```python
from build123d import *

# Parameters (mm, degrees)
EXTRUDE1_DEPTH                                       = 12.7
EXTRUDE2_DEPTH                                       = 3.175
SKETCH3_W                                            = 68.191134733
SKETCH3_H                                            = 44.45
EXTRUDE3_DEPTH                                       = 3.175
SKETCH4_W                                            = 68.191134733
SKETCH4_H                                            = 19.005533376
EXTRUDE4_DEPTH                                       = 3.175
EXTRUDE6_DEPTH                                       = 137.930502446
CBORE_FOR_1_4_BINDING_HEAD_MACHINE_SCREW_D           = 9.525
CBORE_FOR_1_4_BINDING_HEAD_MACHINE_SCREW_CBORE_D     = 17.4752
CBORE_FOR_1_4_BINDING_HEAD_MACHINE_SCREW_CBORE_DEPTH = 3.175
F_7_32_0_21875_DIAMETER_HOLE1_D                      = 5.55625
F_7_32_0_21875_DIAMETER_HOLE1_DEPTH                  = 25.4
F_7_32_0_21875_DIAMETER_HOLE1_TIP                    = 1.669265907
F_7_32_0_21875_DIAMETER_HOLE2_D                      = 5.55625
F_7_32_0_21875_DIAMETER_HOLE2_DEPTH                  = 25.4
F_7_32_0_21875_DIAMETER_HOLE2_TIP                    = 1.669265907


with BuildPart() as part:
    # Sketch1 → Extrude1 (new body)
    with BuildSketch(Plane(origin=(0, 0, 0), x_dir=(1, 0, 0), z_dir=(0, 1, 0))):
        with BuildLine():
            Line((0, 0), (101.6, 0))
            ThreePointArc((101.6, 0), (127, 25.4), (101.6, 50.8))
            Line((101.6, 50.8), (0, 50.8))
            ThreePointArc((0, 50.8), (-24.665230296, 25.4), (0, 0))
        make_face()
    extrude(amount=-EXTRUDE1_DEPTH)

    # Sketch2 → Extrude2 (cut)
    with BuildSketch(Plane(origin=(0, 0, 0), x_dir=(1, 0, 0), z_dir=(0, 1, 0))):
        with BuildLine():
            Line((101.6, 47.625), (0.048151693, 47.625))
            ThreePointArc((0.048151693, 47.625), (-21.490230296, 25.4), (0.048151693, 3.175))
            Line((0.048151693, 3.175), (101.6, 3.175))
            ThreePointArc((101.6, 3.175), (123.825, 25.4), (101.6, 47.625))
        make_face()
    extrude(amount=-EXTRUDE2_DEPTH, mode=Mode.SUBTRACT)

    # Sketch3 → Extrude3 (cut)
    with BuildSketch(Plane(origin=(0, -3.175, 0), x_dir=(-1, 0, 0), z_dir=(0, 1, 0))):
        with Locations((-50.824075847, -25.4)):
            Rectangle(SKETCH3_W, SKETCH3_H)
    extrude(amount=-EXTRUDE3_DEPTH, mode=Mode.SUBTRACT)

    # Sketch4 → Extrude4 (cut)
    with BuildSketch(Plane(origin=(0, -6.35, 0), x_dir=(-1, 0, 0), z_dir=(0, 1, 0))):
        with Locations((-50.824075847, -25.4)):
            Rectangle(SKETCH4_W, SKETCH4_H)
    extrude(amount=-EXTRUDE4_DEPTH, mode=Mode.SUBTRACT)

    # Sketch6 → Extrude6 (cut, through all)
    with BuildSketch(Plane(origin=(0, -6.35, 0), x_dir=(-1, 0, 0), z_dir=(0, 1, 0))):
        with BuildLine():
            Line((-70.286653385, -22.157058497), (-31.585524424, -22.157058497))
            ThreePointArc((-31.585524424, -22.157058497), (-28.07443844, -25.668144481), (-31.585524424, -29.179230465))
            Line((-31.585524424, -29.179230465), (-70.286653385, -29.179230465))
            ThreePointArc((-70.286653385, -29.179230465), (-73.797739369, -25.668144481), (-70.286653385, -22.157058497))
        make_face()
    extrude(amount=-EXTRUDE6_DEPTH, mode=Mode.SUBTRACT)

    # CBORE for 1/4 Binding Head Machine Screw2 (through all)
    with Locations(Plane(origin=(0, -3.175, 0), x_dir=(-1, 0, 0), z_dir=(0, 1, 0))):
        with Locations((-0.745713987, -25.4), (-101.6, -25.4)):
            CounterBoreHole(CBORE_FOR_1_4_BINDING_HEAD_MACHINE_SCREW_D / 2, CBORE_FOR_1_4_BINDING_HEAD_MACHINE_SCREW_CBORE_D / 2, CBORE_FOR_1_4_BINDING_HEAD_MACHINE_SCREW_CBORE_DEPTH)

    # 7/32 (0.21875) Diameter Hole1
    with Locations(Plane(origin=(0, -6.35, 0), x_dir=(-1, 0, 0), z_dir=(0, 1, 0))):
        with Locations((-26.882460023, -9.536116656)):
            Hole(F_7_32_0_21875_DIAMETER_HOLE1_D / 2, depth=F_7_32_0_21875_DIAMETER_HOLE1_DEPTH)
            with Locations((0, 0, -(F_7_32_0_21875_DIAMETER_HOLE1_DEPTH + F_7_32_0_21875_DIAMETER_HOLE1_TIP / 2))):  # 118° drill point
                Cone(0, F_7_32_0_21875_DIAMETER_HOLE1_D / 2, F_7_32_0_21875_DIAMETER_HOLE1_TIP, mode=Mode.SUBTRACT)

    # 7/32 (0.21875) Diameter Hole2
    with Locations(Plane(origin=(0, -6.35, 0), x_dir=(-1, 0, 0), z_dir=(0, 1, 0))):
        with Locations((-50.824075847, -9.536116656), (-74.76569167, -9.536116656), (-26.882460023, -41.263883344), (-50.824075847, -41.263883344), (-74.76569167, -41.263883344)):
            Hole(F_7_32_0_21875_DIAMETER_HOLE2_D / 2, depth=F_7_32_0_21875_DIAMETER_HOLE2_DEPTH)
            with Locations((0, 0, -(F_7_32_0_21875_DIAMETER_HOLE2_DEPTH + F_7_32_0_21875_DIAMETER_HOLE2_TIP / 2))):  # 118° drill point
                Cone(0, F_7_32_0_21875_DIAMETER_HOLE2_D / 2, F_7_32_0_21875_DIAMETER_HOLE2_TIP, mode=Mode.SUBTRACT)


solid = part.part
```
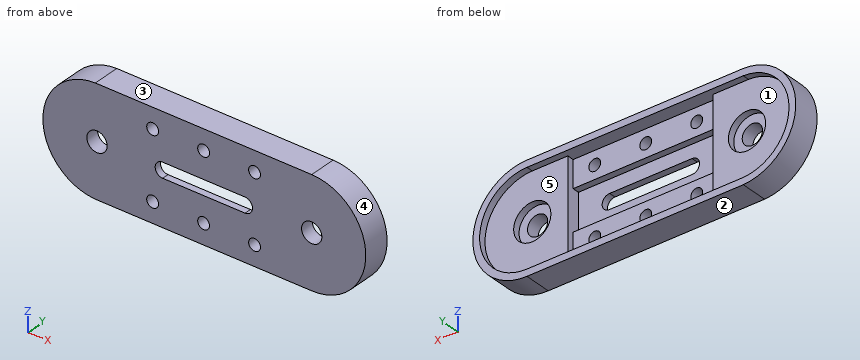
Part model, mm, in its own coordinate system. Face numbers are marked on the shaded views. A direction names the side the tool comes from. Give positions to 0.01 mm unless a question says otherwise; leave off trailing zeros. Order: outer loops, then holes, each group sorted by start corner. A loop starts at its lowest first (then second) coordinate and runs counter-clockwise, first axis right, second up. Notation, with made-up numbers: (68.5, 38) - (72.5, 38) arc R20 cw to (72.5, 65) - close; hole circle Ø7 at (-17, 42). An arc over 180 degrees is marked (long way). Use one line per item in the form item = value.
Item 1: Pin check, flat tips, straight feed: pin 1 Ø3.5 at (x, z) = (26.88, -9.54) entering from +Y; pin 2 Ø9.5 at (x, z) = (54, -28.5) entering from +Y (3 decimals); pin 3 Ø11.5 at (x, z) = (109.5, -36) entering from +Y (3 decimals); pin 4 Ø1.9 at (y, z) = (-7, -19) entering from -X. Stop position of each tip, or through.
Solution:
pin_1 = through
pin_2 = -9.525
pin_3 = -3.175
pin_4 = -24.07
Item 2: Slice it at D-D on x = -2. Give the cut face in (y, z) (3 decimals).
Solution:
outline = (-12.7, -50.662) - (0, -50.662) - (0, -47.466) - (-3.175, -47.466) - (-3.175, -33.695) - (-6.35, -33.695) - (-6.35, -29.291) - (-12.7, -29.291) - close; (-12.7, -21.509) - (-6.35, -21.509) - (-6.35, -17.105) - (-3.175, -17.105) - (-3.175, -3.334) - (0, -3.334) - (0, -0.138) - (-12.7, -0.138) - close
Item 3: Slice it at B-B on y = -4.5. Give the cut face in (x, z) (1 decimal), and give its area (3 significant figures).
Solution:
outline = (0, -50.8) - (101.6, -50.8) arc R25.4 ccw to (101.6, 0) - (0, 0) arc R25.4 ccw to start; hole circle Ø17.5 at (0.7, -25.4); hole (16.7, -47.6) - (84.9, -47.6) - (84.9, -3.2) - (16.7, -3.2) - close; hole circle Ø17.5 at (101.6, -25.4)
area = 3,640 mm2
Item 4: Which spindle directions (+Z, -Z, +X, -X, +Y, -Y) get a long thin tool onto all of the face, cutting with end or side? Do the marked faces 1 and 2. Say none if no direction does.
Solution:
face_1 = +Y
face_2 = -Z, +X, -X, +Y, -Y
Item 5: Slice it at A-A on x = 59.5. Give the cut face in (y, z) (3 decimals), and give its area (3 significant figures).
Solution:
outline = (-12.7, -50.8) - (0, -50.8) - (0, -47.625) - (-6.35, -47.625) - (-6.35, -34.903) - (-9.525, -34.903) - (-9.525, -29.179) - (-12.7, -29.179) - close; (-12.7, -22.157) - (-9.525, -22.157) - (-9.525, -15.897) - (-6.35, -15.897) - (-6.35, -3.175) - (0, -3.175) - (0, 0) - (-12.7, 0) - close
area = 280 mm2
Item 6: Probe probe 1 along Z at (x, y) = (41, -8); probe 2 along Z at (x, y) = (72.5, -10); probe 3 along X at (y, z) = (-7.75, -27). List the from-to ranges inside material, lowest first. Write a range as from..to.
Solution:
probe_1 = -50.8..-34.9, -15.9..0
probe_2 = -50.8..-42.87, -39.66..-28.39, -22.94..-11.14, -7.93..0
probe_3 = -24.61..-3.74, 5.23..16.73, 84.92..97.11, 106.09..126.95
Item 7: Slice it at C-C on z = -25.4. Count the separate pieces of the cut face and the enclosed holes in it, and give its area (3 significant figures).
Solution:
separate_pieces = 4
enclosed_holes = 0
area = 655 mm2
Item 8: Two-plate mould, pull along X, no slides. Class the marked faces 3, 4 and 5: released by +X, released by -X, zero draft, split by the parting line, or undercut.
Solution:
face_3 = zero draft
face_4 = released by +X
face_5 = undercut
